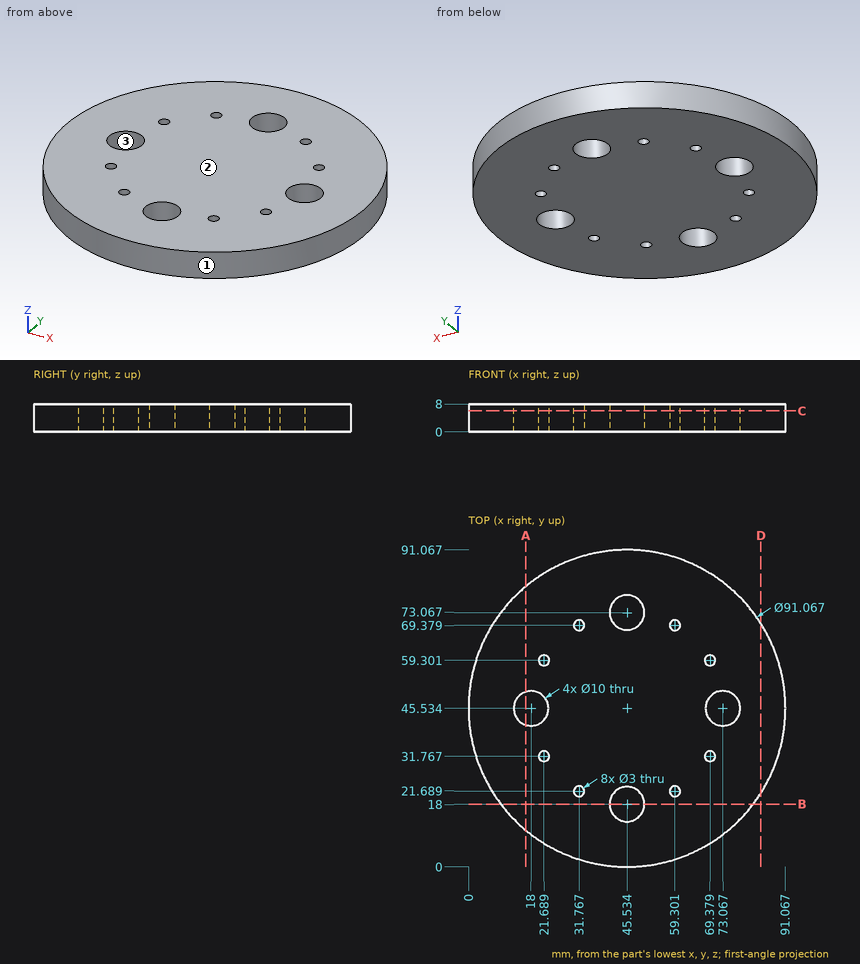
The figure shows three views and two pictorial views of one solid part (mm, origin at its lowest corner). Answer the questions. Coordinates: 2 decimals unless noted, no trailing zeros. Order: outer loops, then holes, each group sorted by start corner. A loop starts at its lowest first (then second) coordinate and runs counter-clockwise, first axis right, second up.
Q1. A cutting plane is placed at C-C, the plane z = 6. State how many separate pieces and enclosed holes the cut face has, and give its area (3 significant figures).
Q2. A cutting plane is placed at D-D, the plane x = 84. Write down the section's boundary in (y, z), and give its area (3 significant figures).
Q3. Consider line 1 (Y direction, x = 33, z = 6.5) (1 decimal); line 2 (X direction, y = 47, z = 0.75) (1 decimal); line 3 (Y direction, x = 32.5, z = 2) (1 decimal). Determine where each line is inside the solid, lowest interval first.
Q4. For a pull along Y with two mould halves and no side action, classify the marked faces 1, 2 and 3 as pulls with the +Y half, pulls with the -Y half, needs draft (parallel to the pull), parting line crosses it, or undercut.
Q5. Given P1, Ø3.5, axis at x = 69.38, y = 59.3, coming from the -Z side; P2, Ø1.8, axis at x = 59.3, y = 69.38, coming from the -Z side; P3, Ø1, axis at x = 40.5, z = 1.5, coming from the +Y side; P4, Ø1, axis at x = 39.5, z = 4, coming from the +Y side, each flat-ended and moving along its own axis, determine where each tip first touches the part or whether it passes through.
Q6. A cutting plane is placed at B-B, the plane y = 18. Write down the section's boundary in (x, z).
Q7. A cutting plane is placed at A-A, the plane x = 16.5. Write down the section's boundary in (y, z), and give its area (3 significant figures).
Answers follow:
1. separate pieces: 1
1. enclosed holes: 12
1. area: 6,140 mm2
2. outline: (21.17, 0) - (69.9, 0) - (69.9, 8) - (21.17, 8) - close
2. area: 390 mm2
3. line 1: y = 1.8 to 20.8, 22.5 to 68.5, 70.2 to 89.3
3. line 2: x = 0 to 13.2, 22.8 to 68.3, 77.8 to 91
3. line 3: y = 1.9 to 20.4, 23 to 68.1, 70.7 to 89.2
4. face 1: parting line crosses it
4. face 2: needs draft
4. face 3: undercut
5. P1: stops at z = 0
5. P2: passes through
5. P3: stops at y = 90.84
5. P4: stops at y = 90.73
6. outline: (9.27, 0) - (40.53, 0) - (40.53, 8) - (9.27, 8) - close; (50.53, 0) - (81.8, 0) - (81.8, 8) - (50.53, 8) - close
7. outline: (10.46, 0) - (40.76, 0) - (40.76, 8) - (10.46, 8) - close; (50.3, 0) - (80.61, 0) - (80.61, 8) - (50.3, 8) - close
7. area: 485 mm2
